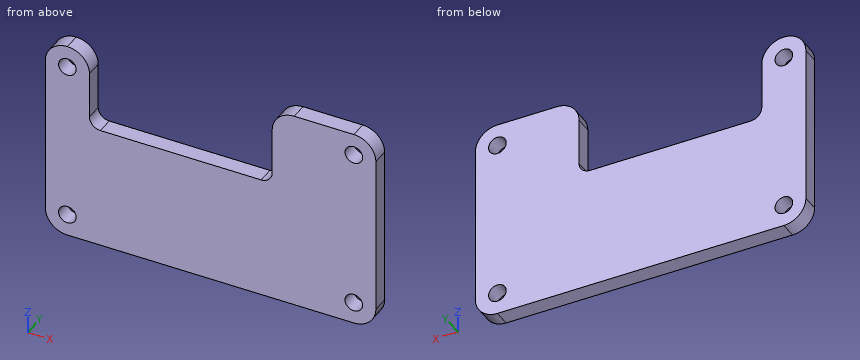
from build123d import *

# Parameters (mm, degrees)
SKETCH1_W           = 60
SKETCH1_H           = 37
BOSS_EXTRUDE1_DEPTH = 2.9972
FILLET1_R           = 4
SKETCH2_R           = 1.6
CUT_EXTRUDE1_DEPTH  = 36.372774952
SKETCH3_W           = 33.176
SKETCH3_H           = 14.5
CUT_EXTRUDE2_DEPTH  = 36.372774952
FILLET2_R           = 4
FILLET3_R           = 2


with BuildPart() as part:
    # Sketch1 → Boss-Extrude1 (new body)
    with BuildSketch(Plane(origin=(0, 0, 0), x_dir=(1, 0, 0), z_dir=(0, 1, 0))):
        Rectangle(SKETCH1_W, SKETCH1_H)
    extrude(amount=BOSS_EXTRUDE1_DEPTH)

    # Fillet1
    fillet1_edges = [part.edges().sort_by_distance(p)[0] for p in [
        (30, 1.4986, 18.5),
        (-30, 1.4986, 18.5),
        (-30, 1.4986, -18.5),
        (30, 1.4986, -18.5),
    ]]
    fillet(fillet1_edges, radius=FILLET1_R)

    # Sketch2 → Cut-Extrude1 (cut, through all)
    with BuildSketch(Plane(origin=(0, 2.9972, 0), x_dir=(1, 0, 0), z_dir=(0, 1, 0))):
        with Locations(Location((-26, 14.5, 0), (0, 0, 270))):
            Circle(SKETCH2_R)
        with Locations(Location((-26, -14.5, 0), (0, 0, 270))):
            Circle(SKETCH2_R)
        with Locations(Location((26, -14.5, 0), (0, 0, 270))):
            Circle(SKETCH2_R)
        with Locations(Location((26, 14.5, 0), (0, 0, 270))):
            Circle(SKETCH2_R)
    extrude(amount=-CUT_EXTRUDE1_DEPTH, mode=Mode.SUBTRACT)

    # Sketch3 → Cut-Extrude2 (cut, through all)
    with BuildSketch(Plane(origin=(0, 2.9972, 0), x_dir=(1, 0, 0), z_dir=(0, 1, 0))):
        with Locations((-5.412, -11.25)):
            Rectangle(SKETCH3_W, SKETCH3_H)
    extrude(amount=-CUT_EXTRUDE2_DEPTH, mode=Mode.SUBTRACT)

    # Fillet2
    fillet2_edges = [part.edges().sort_by_distance(p)[0] for p in [
        (11.176, 1.4986, 18.5),
        (-22, 1.4986, 18.5),
    ]]
    fillet(fillet2_edges, radius=FILLET2_R - 0.0001)  # a hair under: the kernel refuses the full size

    # Fillet3
    fillet3_edges = [part.edges().sort_by_distance(p)[0] for p in [
        (11.176, 1.4986, 4),
        (-22, 1.4986, 4),
    ]]
    fillet(fillet3_edges, radius=FILLET3_R)


solid = part.part
Build history of the part. All positions in model axes, mm. Round coordinates to 2 decimals unless told otherwise and drop trailing zeros. Write each loop counter-clockwise with the first axis right and the second up, starting at its lowest first coordinate (ties: lowest second). Pieces come first, ordered by that corner, then holes. Notation, with made-up numbers: M 70,-30 L 105,-30 A10 ccw 105,-13 Z; hole C 51.25,-16 d6. An arc over 180 degrees is marked long. Answer as a JSON object with one key per item and string values. Group by question number.
(1) Cut at B-B (y = 0.9). Give the number of separate pieces and of enclosed holes in the cut face, and give its area (3 significant figures).
(2) Drill centre lines: L1, parallel to X at y = 0.7, z = -14.5; L2, parallel to X at y = 2.2, z = 14.5; L3, parallel to X at y = 0.3, z = 6. Where is each one in solid material? Low to high.
(3) Cut at C-C (x = -6). Give the cut face in (y, z), and give its area (3 significant figures).
(4) Cut at A-A (z = 8.5). Give the cut face in (x, y).
(5) Flat gauge pin, fed straight in: pin 1 (1 mm diameter, centred on x = -10.5, z = -13.5, fed in from -Y). Where does the tip first touch, or does it go through?
Responses:
{
 "1": {"separate pieces": "1", "enclosed holes": "4", "area": "1,690 mm2"},
 "2": {"L1": "x = -30 to -27.6, -24.4 to 24.4, 27.6 to 30", "L2": "x = -30 to -27.6, -24.4 to -22, 11.18 to 24.4, 27.6 to 30", "L3": "x = -30 to -22, 11.18 to 30"},
 "3": {"outline": "M 0,-18.5 L 3,-18.5 L 3,4 L 0,4 Z", "area": "67.4 mm2"},
 "4": {"outline": "M -30,0 L -22,0 L -22,3 L -30,3 Z; M 11.18,0 L 30,0 L 30,3 L 11.18,3 Z"},
 "5": {"pin 1": "stops at y = 0"}
}
